from build123d import *

# Parameters (mm, degrees)
SKETCH1_W                      = 300
SKETCH1_H                      = 450
BOSS_EXTRUDE1_DEPTH            = 80
SHELL1_T                       = -10
SKETCH2_W                      = 30
SKETCH2_H                      = 30
BOSS_EXTRUDE2_DEPTH            = 15
BOSS_EXTRUDE4_REACH            = 366.211
SKETCH3_R                      = 4
SKETCH4_R                      = 4
BOSS_EXTRUDE5_DEPTH            = 250
BOSS_EXTRUDE6_DEPTH            = 210
BOSS_EXTRUDE6_DEPTH_BACK       = 80
SKETCH5_W                      = 25
SKETCH5_H                      = 40
SKETCH6_W                      = 35
SKETCH6_H                      = 80
CUT_EXTRUDE1_DEPTH             = 300
BOSS_EXTRUDE7_START            = -80
SKETCH8_W                      = 25
SKETCH8_H                      = 40
BOSS_EXTRUDE7_DEPTH            = 290
CUT_EXTRUDE2_REACH             = 460.639
SKETCH10_R                     = 5
CUT_EXTRUDE2_DIRECTION_2_DEPTH = 300


with BuildPart() as part:
    # Sketch1 → Boss-Extrude1 (new body)
    with BuildSketch(Plane(origin=(0, 0, 0), x_dir=(1, 0, 0), z_dir=(0, 1, 0))):
        Rectangle(SKETCH1_W, SKETCH1_H)
    extrude(amount=BOSS_EXTRUDE1_DEPTH)

    # Shell1
    shell1_openings = [part.faces().sort_by_distance(p)[0] for p in [
        (0, 80, 0),
        (0, 0, 0),
    ]]
    offset(amount=SHELL1_T, openings=shell1_openings, kind=Kind.INTERSECTION)

    # Sketch2 → Boss-Extrude2 (add)
    with BuildSketch(Plane.ZY.offset(-140)):
        with Locations((-200, 15)):
            Rectangle(SKETCH2_W, SKETCH2_H)
        with Locations((200, 57.274341307)):
            Rectangle(SKETCH2_W, SKETCH2_H)
    boss_extrude2 = extrude(amount=BOSS_EXTRUDE2_DEPTH)

    # Mirror2: Boss-Extrude2 across plane
    add(boss_extrude2.mirror(Plane(origin=(0, 0, 0), x_dir=(0, 0, 1), z_dir=(1, 0, 0))))

    # Sketch3 → Boss-Extrude4 (add, up to next)
    with BuildSketch(Plane.ZY.offset(-125), mode=Mode.PRIVATE) as boss_extrude4_sk1:
        with Locations(Location((-200, 15, 0), (0, 0, 180))):
            Circle(SKETCH3_R)
    boss_extrude4_tool1 = extrude(boss_extrude4_sk1.sketch, amount=BOSS_EXTRUDE4_REACH, mode=Mode.PRIVATE) - part.part
    add(boss_extrude4_tool1.solids().sort_by_distance((125, 15, -200))[0])

    # Sketch4 → Boss-Extrude5 (add)
    with BuildSketch(Plane.ZY.offset(-125)):
        with Locations(Location((200, 57.274341307, 0), (0, 0, 180))):
            Circle(SKETCH4_R)
    extrude(amount=BOSS_EXTRUDE5_DEPTH)

    # Sketch5 → Boss-Extrude6 (add, two sides: drawn at the far end of the back side and taken through both)
    with BuildSketch(Plane(origin=(0, 80, 0), x_dir=(1, 0, 0), z_dir=(0, 1, 0)).offset(-BOSS_EXTRUDE6_DEPTH_BACK)):
        with Locations((137.5, 205)):
            Rectangle(SKETCH5_W, SKETCH5_H)
    extrude(amount=BOSS_EXTRUDE6_DEPTH + BOSS_EXTRUDE6_DEPTH_BACK)

    # Sketch6 → Cut-Extrude1 (cut)
    with BuildSketch(Plane.XY.offset(-215)):
        with Locations((107.5, 40)):
            Rectangle(SKETCH6_W, SKETCH6_H)
    extrude(amount=-CUT_EXTRUDE1_DEPTH, mode=Mode.SUBTRACT)

    # Sketch8 → Boss-Extrude7 (add)
    with BuildSketch(Plane(origin=(0, 80, 0), x_dir=(1, 0, 0), z_dir=(0, 1, 0)).offset(BOSS_EXTRUDE7_START)):
        with Locations((77.5, 205)):
            Rectangle(SKETCH8_W, SKETCH8_H)
    extrude(amount=BOSS_EXTRUDE7_DEPTH)

    # Cut-Extrude2: up to this face of the body (flat: up to its plane)
    cut_extrude2_end = Plane(part.part.faces().sort_by_distance((65, 153.422023127, -203.907073233))[0])
    # Sketch10 → Cut-Extrude2 (cut, up to the picked face)
    with BuildSketch(Plane.ZY.offset(-125), mode=Mode.PRIVATE) as cut_extrude2_sk1:
        with Locations((-205, 270)):
            Circle(SKETCH10_R)
    cut_extrude2_tool1 = split(extrude(cut_extrude2_sk1.sketch, amount=CUT_EXTRUDE2_REACH, mode=Mode.PRIVATE), bisect_by=cut_extrude2_end, keep=Keep.BOTH, mode=Mode.PRIVATE)
    add(cut_extrude2_tool1.solids().sort_by(Axis((125, 270, -205), (-1, 0, 0)))[0], mode=Mode.SUBTRACT)

    # Sketch10 → Cut-Extrude2 direction 2 (cut)
    with BuildSketch(Plane.ZY.offset(-125)):
        with Locations((-205, 270)):
            Circle(SKETCH10_R)
    extrude(amount=-CUT_EXTRUDE2_DIRECTION_2_DEPTH, mode=Mode.SUBTRACT)


solid = part.part
Input: part model. Units: mm. Frame: model coordinates. A direction names the side the tool comes from. Give positions to 0.01 mm unless a question says otherwise; leave off trailing zeros. Loops run counter-clockwise (first coordinate to the right, second up) from the corner with the lowest first, then second, coordinate; pieces in that order, holes last. Notation, with made-up numbers: (-17.5, -20.75) -> (-0.5, -20.75) arc R20 ccw to (-0.5, -16.75) -> close; hole circle Ø7 at (-16.75, -14). An arc over 180 degrees is marked (long way). Answer as a JSON object with one key per item and string values. Group by question number.
Item 1: Cut plane C-C, the plane y = 270. Return the cut outline in (x, z).
Item 2: Cut plane D-D, the plane x = 12.5. Return the cut outline in (y, z), and give its area (3 significant figures).
Item 3: Line query: probe 1 along Z at (x, y) = (137, 270); probe 2 along Y at (x, z) = (72, -205); probe 3 along Z at (x, y) = (133, 19.5). Output: solid intervals per line, ascending.
Item 4: Reachability of faces 4 (the flat face through (-133, 57, 185)), 5 (the cylindrical face through (78, 274, -202)), 6 (the flat face through (-133, 30, -200)), 7 (the flat face through (-125, 12, -197)), 8 (the flat face through (133, 42.274, 200)) from +Z, -Z, +X, -X, +Y, -Y: full face, straight path, thin tool, end or side. Return the list, or none.
Item 5: Pull-direction query (X, two-part tool) for faces 1 (the flat face through (-2, 39, 225)), 2 (the flat face through (-140, 39, 3)), 3 (the flat face through (-150, 39, 3)); classes: released by +X, released by -X, zero draft, split by the parting line, or undercut.
Item 6: Cut plane B-B, the plane y = 187. Return the cut outline in (x, z).
Item 7: Cut plane A-A, the plane z = 45. Return the cut outline in (x, y), and give its area (3 significant figures).
Item 8: Pin query (flat end, axial travel): P1, Ø20, axis at y = 116.5, z = -214.5, coming from the -X side; P2, Ø12, axis at x = -130.5, z = 206.5, coming from the -Y side; P3, Ø16.5, axis at x = 131.5, z = 203, coming from the +Y side. Return the tip coordinate at first contact, or that it passes through.
Checks:
{
 "1": {"outline": "(65, -225) -> (90, -225) -> (90, -210) -> (65, -210) -> close; (65, -200) -> (90, -200) -> (90, -185) -> (65, -185) -> close; (125, -225) -> (150, -225) -> (150, -210) -> (125, -210) -> close; (125, -200) -> (150, -200) -> (150, -185) -> (125, -185) -> close"},
 "2": {"outline": "(0, -225) -> (80, -225) -> (80, -215) -> (0, -215) -> close; (0, 215) -> (80, 215) -> (80, 225) -> (0, 225) -> close; circle Ø8 at (15, -200); circle Ø8 at (57.27, 200)", "area": "1,700 mm²"},
 "3": {"probe 1": "z = -225 to -210, -200 to -185", "probe 2": "y = 0 to 265, 275 to 290", "probe 3": "z = -225 to -185, 215 to 225"},
 "4": {"face 4": "+Y, -Y", "face 5": "+X, -X", "face 6": "+Y", "face 7": "none", "face 8": "-Y"},
 "5": {"face 1": "zero draft", "face 2": "undercut", "face 3": "released by -X"},
 "6": {"outline": "(65, -225) -> (90, -225) -> (90, -185) -> (65, -185) -> close; (125, -225) -> (150, -225) -> (150, -185) -> (125, -185) -> close"},
 "7": {"outline": "(-150, 0) -> (-140, 0) -> (-140, 80) -> (-150, 80) -> close; (140, 0) -> (150, 0) -> (150, 80) -> (140, 80) -> close", "area": "1,600 mm²"},
 "8": {"P1": "stops at x = 65", "P2": "stops at y = 42.27", "P3": "stops at y = 72.27"}
}
